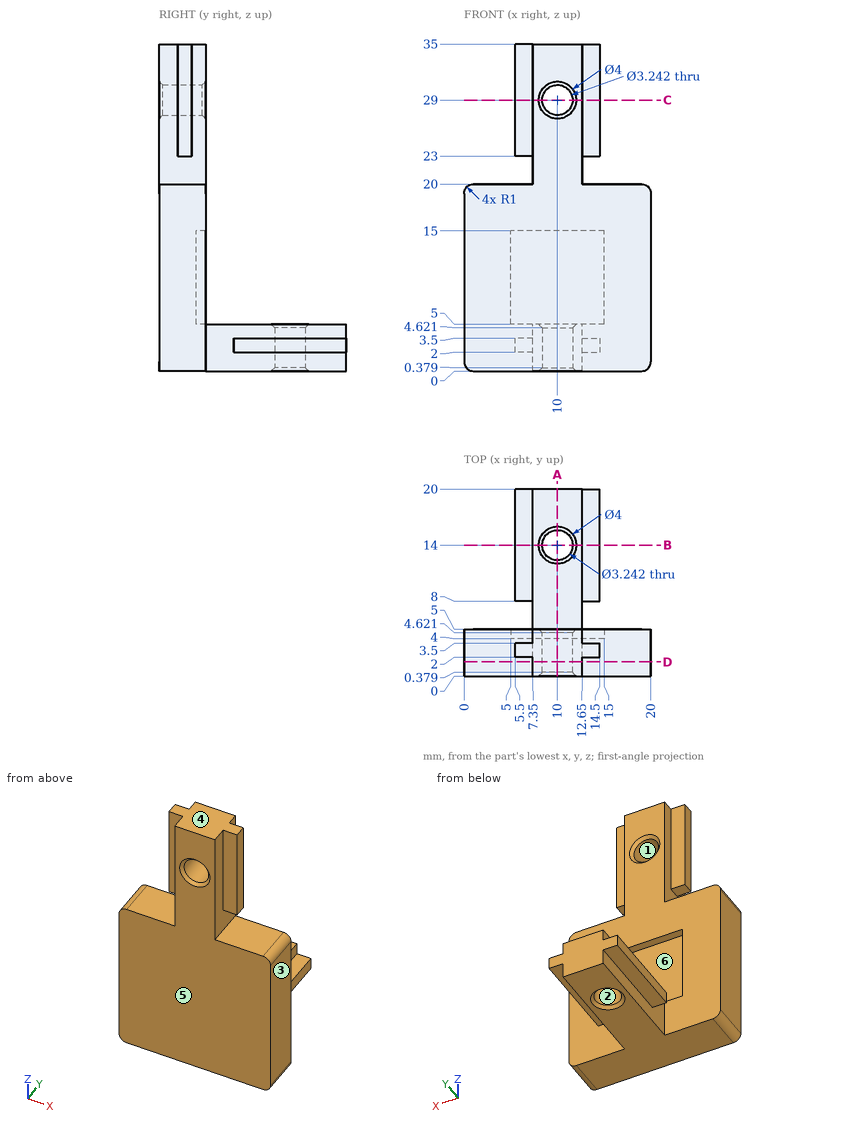
Part print with two shaded views. Sizes in mm from the minimum x, y, z corner. A direction names the side the tool comes from. Give positions to 0.01 mm unless a question says otherwise; leave off trailing zeros. Order: outer loops, then holes, each group sorted by start corner. A loop starts at its lowest first (then second) coordinate and runs counter-clockwise, first axis right, second up. Notation, with made-up numbers: M 11.25,40.25 L 52.25,40.25 A23 ccw 52.25,60.25 Z; hole C 71.5,-24.5 d4. An arc over 180 degrees is marked long. Put each result on its own line as item: value.
Item 1: Which spindle directions (+Z, -Z, +X, -X, +Y, -Y) get a long thin tool onto all of the face, cutting with end or side? Do the marked faces 5 and 6. Say none if no direction does.
Results are:
face 5: +Z, -Z, +X, -X, -Y
face 6: +Y
Item 2: Wall check: probe 1 along Y at (x, z) = (10, 1.5); probe 2 along Z at (x, y) = (10, 2.7); probe 3 along X at (y, z) = (1.25, 29). Give the ranges that are in metal, low to high.
Results are:
probe 1: 0 to 12.38, 15.62 to 20
probe 2: 0 to 27.38, 30.62 to 35
probe 3: 7.35 to 8.38, 11.62 to 12.65
Item 3: Pull direction X, two halves, no side cores. Call the marked faces 1, 2, 3 and 4: +X half, -X half, draft (parallel to the pull), parting line (faces both ways), or undercut.
Results are:
face 1: undercut
face 2: undercut
face 3: +X half
face 4: draft
Item 4: Cut at A-A on x = 10. Write the cut outline in (y, z), then the cut area to 3 significant figures.
Results are:
outline: M 0,0 L 12,0 L 12.38,0.38 L 12.38,4.62 L 12,5 L 4,5 L 4,15 L 5,15 L 5,27 L 4.62,27.38 L 0.38,27.38 L 0,27 Z; M 0,31 L 0.38,30.62 L 4.62,30.62 L 5,31 L 5,35 L 0,35 Z; M 15.62,0.38 L 16,0 L 20,0 L 20,5 L 16,5 L 15.62,4.62 Z
area: 207 mm2
Item 5: Drop flat-ended pins along their axis: pin 1 Ø2 at (x, y) = (6.5, 10) entering from +Z; pin 2 Ø0.8 at (y, z) = (13.5, 3) entering from +X; pin 3 Ø4 at (y, z) = (1.5, 29.5) entering from -X. Give the stop position or say it passes through.
Results are:
pin 1: z = 5
pin 2: x = 14.5
pin 3: x = 5.5
Item 6: Cut at D-D on y = 1.5. Write the cut outline in (x, z), then the cut area to 3 significant figures.
Results are:
outline: M 0,1 A1 ccw 1,0 L 19,0 A1 ccw 20,1 L 20,19 A1 ccw 19,20 L 12.65,20 L 12.65,35 L 7.35,35 L 7.35,20 L 1,20 A1 ccw 0,19 Z; hole C 10,29 d3.24
area: 470 mm2
Item 7: Cut at B-B on y = 14. Write the cut outline in (x, z), then the cut area to 3 significant figures.
Results are:
outline: M 5.5,2 L 7.35,2 L 7.35,0 L 8,0 L 8.38,0.38 L 8.38,4.62 L 8,5 L 7.35,5 L 7.35,3.5 L 5.5,3.5 Z; M 11.62,0.38 L 12,0 L 12.65,0 L 12.65,2 L 14.5,2 L 14.5,3.5 L 12.65,3.5 L 12.65,5 L 12,5 L 11.62,4.62 Z
area: 15.6 mm2
